Input: part model. Units: mm. Frame: model coordinates. Face numbers are marked on the shaded views. A direction names the side the tool comes from. Coordinates: 2 decimals unless noted, no trailing zeros. Write each loop counter-clockwise with the first axis right and the second up, starting at its lowest first coordinate (ties: lowest second). Pieces come first, ordered by that corner, then holes. Notation, with made-up numbers: (0, 30) -> (28, 30) arc R37 ccw to (28, 68) -> close; hole circle Ø6 at (-16, 88). An arc over 180 degrees is marked (long way). Use one line per item in the form item = value. Start each with the question number.
(1) Cut plane B-B on x = 11. Return the cut outline in (y, z).
(2) Set-up query: the marked faces 3 and 4. Return all of +Z, -Z, +X, -X, +Y, -Y with unobstructed straight access to the full face (end or side cutting, diameter ignored); none if empty.
(3) Cut plane A-A on z = 2.35. State how many separate pieces and enclosed holes the cut face has, plus the area to 3 significant figures.
(4) Cut plane C-C on x = 4. Return the cut outline in (y, z), plus the area to 3 significant figures.
(5) Ray query, line 1 along Y through (x, z) = (0, 4.2); line 2 along Y through (x, z) = (1.75, 2.35); line 3 along Y through (x, z) = (-9.5, 4.15). Return the intervals inside material, ascending.
(6) First-contact query: pin 1 (2.5 mm diameter, centred on y = -61, z = 3, fed in from +X); pin 2 (2.5 mm diameter, centred on y = -103.5, z = 2, fed in from +X); pin 3 (1.6 mm diameter, centred on y = -24, z = 2, fed in from -X). Flat tips, straight axial feed; report the tip coordinate or a pass-through.
(7) Pull-direction query (X, two-part tool) for the marked faces 1 and 2; classes: released by +X, released by -X, zero draft, split by the parting line, or undercut.
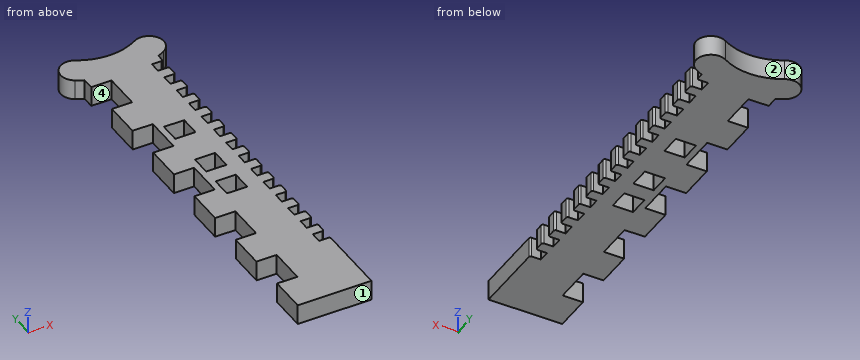
```python
from build123d import *

# Parameters (mm, degrees)
EXTRUDE_1_DEPTH     = 5.5
SKETCH_2_W          = 5.5
SKETCH_2_H          = 10
SKETCH_2_W_2        = 3
SKETCH_2_H_2        = 3
CUT_EXTRUDE_1_DEPTH = 126.901747406
SKETCH_5_W          = 5.5
SKETCH_5_H          = 5.5
CUT_EXTRUDE_2_DEPTH = 126.901747406
FILLET_1_R          = 0.5


with BuildPart() as part:
    # ｽｹｯﾁ1 → ﾎﾞｽ - 押し出し1 (new body)
    with BuildSketch(Plane.XY):
        with BuildLine():
            Line((-10, -21.817424229), (-10, -125))
            Line((-10, -125), (10, -125))
            Line((10, -125), (10, -21.817424229))
            ThreePointArc((10, -21.817424229), (11.012114986, -21.324477099), (12, -20.784609691))
            ThreePointArc((12, -20.784609691), (13.464101615, -15.320508076), (8, -13.856406461))
            ThreePointArc((8, -13.856406461), (0, -16), (-8, -13.856406461))
            ThreePointArc((-8, -13.856406461), (-13.464101615, -15.320508076), (-12, -20.784609691))
            ThreePointArc((-12, -20.784609691), (-11.012114986, -21.324477099), (-10, -21.817424229))
        make_face()
    extrude(amount=EXTRUDE_1_DEPTH)

    # ｽｹｯﾁ2 → ｶｯﾄ - 押し出し1 (cut, through all)
    with BuildSketch(Plane.XY.offset(5.5)):
        with Locations((-7.25, -90)):
            Rectangle(SKETCH_2_W, SKETCH_2_H)
        with Locations((-7.25, -110)):
            Rectangle(SKETCH_2_W, SKETCH_2_H)
        with Locations((-7.25, -70)):
            Rectangle(SKETCH_2_W, SKETCH_2_H)
        with Locations((-7.25, -50)):
            Rectangle(SKETCH_2_W, SKETCH_2_H)
        with Locations((-7.25, -30)):
            Rectangle(SKETCH_2_W, SKETCH_2_H)
        with Locations((8.5, -103.5)):
            Rectangle(SKETCH_2_W_2, SKETCH_2_H_2)
        with Locations((8.5, -97.5)):
            Rectangle(SKETCH_2_W_2, SKETCH_2_H_2)
        with Locations((8.5, -91.5)):
            Rectangle(SKETCH_2_W_2, SKETCH_2_H_2)
        with Locations((8.5, -85.5)):
            Rectangle(SKETCH_2_W_2, SKETCH_2_H_2)
        with Locations((8.5, -79.5)):
            Rectangle(SKETCH_2_W_2, SKETCH_2_H_2)
        with Locations((8.5, -73.5)):
            Rectangle(SKETCH_2_W_2, SKETCH_2_H_2)
        with Locations((8.5, -67.5)):
            Rectangle(SKETCH_2_W_2, SKETCH_2_H_2)
        with Locations((8.5, -61.5)):
            Rectangle(SKETCH_2_W_2, SKETCH_2_H_2)
        with Locations((8.5, -55.5)):
            Rectangle(SKETCH_2_W_2, SKETCH_2_H_2)
        with Locations((8.5, -49.5)):
            Rectangle(SKETCH_2_W_2, SKETCH_2_H_2)
        with Locations((8.5, -43.5)):
            Rectangle(SKETCH_2_W_2, SKETCH_2_H_2)
        with Locations((8.5, -37.5)):
            Rectangle(SKETCH_2_W_2, SKETCH_2_H_2)
        with Locations((8.5, -31.5)):
            Rectangle(SKETCH_2_W_2, SKETCH_2_H_2)
        with Locations((8.5, -25.5)):
            Rectangle(SKETCH_2_W_2, SKETCH_2_H_2)
    extrude(amount=-CUT_EXTRUDE_1_DEPTH, mode=Mode.SUBTRACT)

    # ｽｹｯﾁ5 → ｶｯﾄ - 押し出し2 (cut, through all)
    with BuildSketch(Plane.XY.offset(5.5)):
        with Locations((0, -65)):
            Rectangle(SKETCH_5_W, SKETCH_5_H)
        with Locations((0, -50)):
            Rectangle(SKETCH_5_W, SKETCH_5_H)
        with Locations((0, -75)):
            Rectangle(SKETCH_5_W, SKETCH_5_H)
    extrude(amount=-CUT_EXTRUDE_2_DEPTH, mode=Mode.SUBTRACT)

    # ﾌｨﾚｯﾄ1
    fillet_1_edges = [part.edges().sort_by_distance(p)[0] for p in [
        (10, -39, 2.75),
        (10, -36, 2.75),
        (10, -45, 2.75),
        (10, -42, 2.75),
        (10, -51, 2.75),
        (10, -48, 2.75),
        (10, -57, 2.75),
        (10, -54, 2.75),
        (10, -63, 2.75),
        (10, -60, 2.75),
        (10, -69, 2.75),
        (10, -66, 2.75),
        (10, -75, 2.75),
        (10, -72, 2.75),
        (10, -81, 2.75),
        (10, -78, 2.75),
        (10, -87, 2.75),
        (10, -84, 2.75),
        (10, -93, 2.75),
        (10, -90, 2.75),
        (10, -99, 2.75),
        (10, -96, 2.75),
        (10, -102, 2.75),
        (10, -105, 2.75),
        (10, -33, 2.75),
        (10, -30, 2.75),
        (10, -27, 2.75),
        (10, -24, 2.75),
    ]]
    fillet(fillet_1_edges, radius=FILLET_1_R)


solid = part.part
```
Values:
q1.outline = (-21.33, 0) -> (-13.45, 0) -> (-13.45, 5.5) -> (-21.33, 5.5) -> close
q2.face_3 = +Z, -Z
q2.face_4 = +Z, -Z, -X
q3.separate_pieces = 1
q3.enclosed_holes = 3
q3.area = 1,760 mm2
q4.outline = (-125, 0) -> (-15.49, 0) -> (-15.49, 5.5) -> (-125, 5.5) -> close
q4.area = 602 mm2
q5.line_1 = -125 to -77.75, -72.25 to -67.75, -62.25 to -52.75, -47.25 to -16
q5.line_2 = -125 to -77.75, -72.25 to -67.75, -62.25 to -52.75, -47.25 to -15.9
q5.line_3 = -125 to -115, -105 to -95, -85 to -75, -65 to -55, -45 to -35, -25 to -13.35
q6.pin_1 = 9.93
q6.pin_2 = 7
q6.pin_3 = -10
q7.face_1 = zero draft
q7.face_2 = undercut
